The model under review builds one solid part; all positions refer to its coordinate system, in mm. Face numbers are marked on the shaded views. A direction names the side the tool comes from. Give positions to 0.01 mm unless a question says otherwise; leave off trailing zeros. Order: outer loops, then holes, each group sorted by start corner. A loop starts at its lowest first (then second) coordinate and runs counter-clockwise, first axis right, second up. Notation, with made-up numbers: (79.25, -13) - (137.25, -13) arc R24 cw to (137.25, 10) - close; hole circle Ø6 at (51, -20). An arc over 180 degrees is marked (long way). Use CSV: the item, a comma, the result in double quotes.
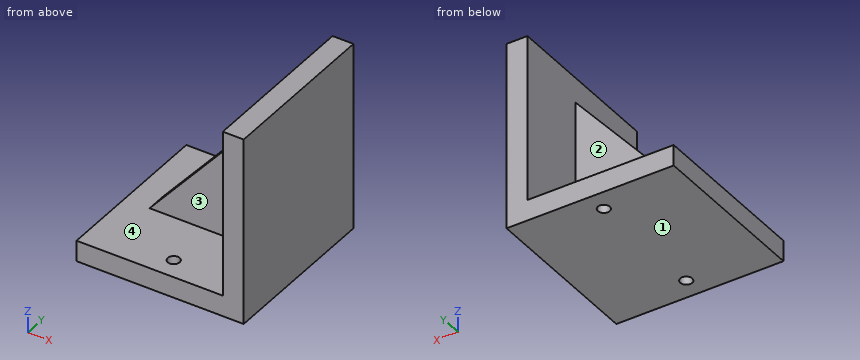
```python
from build123d import *

# Parameters (mm, degrees)
F1_DEPTH = 25.4
F2_DEPTH = 3.175
F3_R     = 1.811143
F4_DEPTH = 25.4


with BuildPart() as f1:
    # F0 (on Front) → F1 (new body, symmetric)
    with BuildSketch(Plane.XZ):
        Polygon((-38.864661, 19.945657), (-46.484661, 19.945657), (-46.484661, 13.595657), (4.315339, 13.595657), (4.315339, 19.945657), (-2.034661, 19.945657), align=None)
        Polygon((-2.034661, 63.125657), (-2.034661, 19.945657), (4.315339, 19.945657), (4.315339, 70.745657), (-2.034661, 70.745657), align=None)
    extrude(amount=F1_DEPTH, both=True)

    # F0 (on Front) → F2 (join, symmetric)
    with BuildSketch(Plane.XZ):
        Polygon((-38.864661, 19.945657), (-46.484661, 19.945657), (-46.484661, 13.595657), (4.315339, 13.595657), (4.315339, 19.945657), (-2.034661, 19.945657), align=None)
        Polygon((-2.034661, 63.125657), (-38.864661, 19.945657), (-2.034661, 19.945657), align=None)
        Polygon((-2.034661, 63.125657), (-2.034661, 19.945657), (4.315339, 19.945657), (4.315339, 70.745657), (-2.034661, 70.745657), align=None)
    extrude(amount=F2_DEPTH, both=True)

    # F3 (on face) → F4 (cut)
    with BuildSketch(Plane.XY.offset(19.945657)):
        with Locations((-21.084661, 19.05)):
            Circle(F3_R)
        with Locations((-21.115254, -19.049988)):
            Circle(F3_R)
    extrude(amount=-F4_DEPTH, mode=Mode.SUBTRACT)


solid = f1.part
```
Item 1: Wall thickness on L1, parallel to X at y = 19, z = 18; L2, parallel to Z at x = -33, y = -6; L3, parallel to X at y = -7.5, z = 39.5: over which ranges is each line inside the solid? List them lowest first.
Results list:
L1,"x = -46.48 to -22.9, -19.27 to 4.32"
L2,"z = 13.6 to 19.95"
L3,"x = -2.03 to 4.32"
Item 2: Take a section at B-B, the plane y = -8.5. Give the boundary of the cut face in (x, z).
Results list:
outline,"(-46.48, 13.6) - (4.32, 13.6) - (4.32, 70.75) - (-2.03, 70.75) - (-2.03, 19.95) - (-46.48, 19.95) - close"
Item 3: Take a section at A-A, the plane y = 19.05. Give the boundary of the cut face in (x, z).
Results list:
outline,"(-46.48, 13.6) - (-22.9, 13.6) - (-22.9, 19.95) - (-46.48, 19.95) - close; (-19.27, 13.6) - (4.32, 13.6) - (4.32, 70.75) - (-2.03, 70.75) - (-2.03, 19.95) - (-19.27, 19.95) - close"
Item 4: Take a section at D-D, the plane z = 37.5. Give the boundary of the cut face in (x, y) (3 decimals).
Results list:
outline,"(-23.892, -3.175) - (-2.035, -3.175) - (-2.035, -25.4) - (4.315, -25.4) - (4.315, 25.4) - (-2.035, 25.4) - (-2.035, 3.175) - (-23.892, 3.175) - close"
Item 5: Take a section at C-C, the plane x = -6.5. Give the boundary of the cut face in (y, z) (3 decimals), and give its area (3 significant figures).
Results list:
outline,"(-25.4, 13.596) - (25.4, 13.596) - (25.4, 19.946) - (3.175, 19.946) - (3.175, 57.89) - (-3.175, 57.89) - (-3.175, 19.946) - (-25.4, 19.946) - close"
area,"564 mm2"
Item 6: Tool access review of the marked faces 1, 2, 3 and 4: name each direction out of +Z, -Z, +X, -X, +Y, -Y from which nothing blocks a thin tool from reaching the whole face with its end or side.
Results list:
face 1,"-Z, +X, -X, +Y, -Y"
face 2,"+Z, -X, +Y"
face 3,"+Z, -X, -Y"
face 4,"+Z, -X"
Item 7: Clearance check with flat-ended pins moving along their axes: pin 1 (1 mm diameter, centred on y = 12.5, z = 30, fed in from -X); pin 2 (22 mm diameter, centred on x = -30.5, y = 2.5, fed in from +Z); pin 3 (11 mm diameter, centred on x = -13.5, z = 36.5, fed in from +Y) (3 decimals); pin 4 (2 mm diameter, centred on x = -21.12, y = -19.05, fed in from +Z). State where each tip first meets the part, or that it passes through.
Results list:
pin 1,"stops at x = -2.03"
pin 2,"stops at z = 42.65"
pin 3,"stops at y = 3.175"
pin 4,"passes through"
